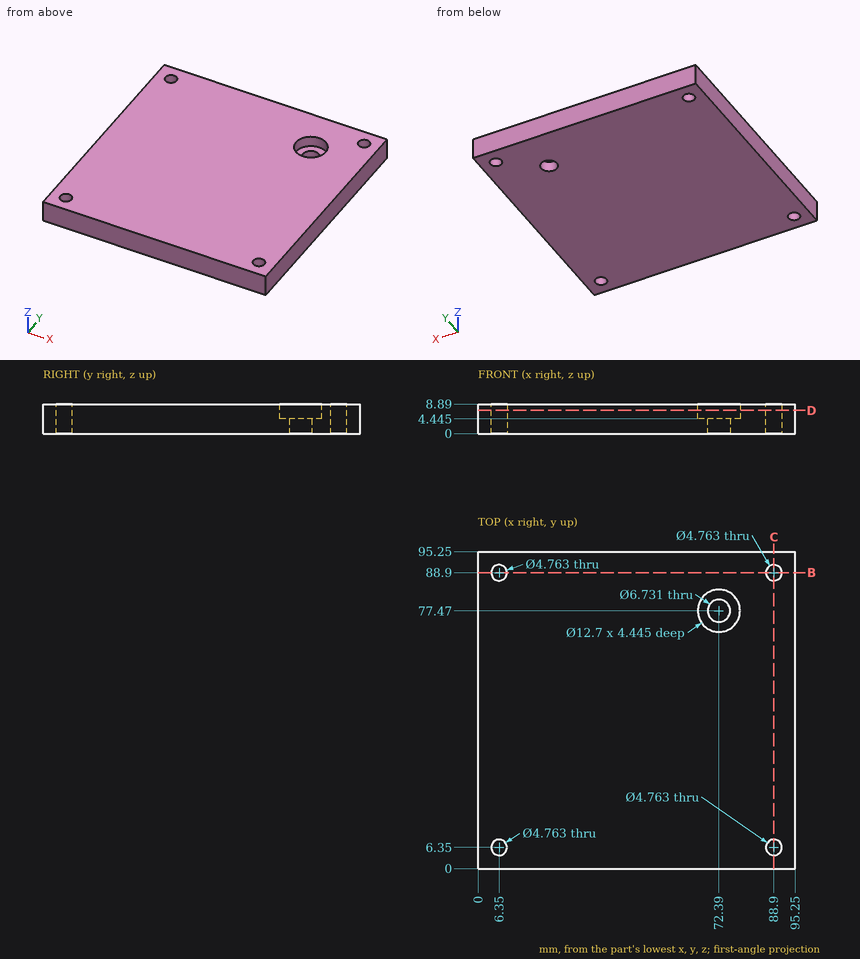
Source: three-view drawing plus pictorial views. Frame: mm from the lowest corner of the part. Coordinates: 2 decimals unless noted, no trailing zeros. Loops run counter-clockwise (first coordinate to the right, second up) from the corner with the lowest first, then second, coordinate; pieces in that order, holes last. Notation, with made-up numbers: (-13.5, 71) - (7.5, 71) arc R23 cw to (7.5, 96) - close; hole circle Ø6 at (-22.75, 4.25). An arc over 180 degrees is marked (long way). One line per item, written item: value. Start each with the question number.
1. Section B-B (y = 88.9). Return the cut outline in (x, z).
2. Ray query, L1, parallel to Y at x = 88.9, z = 7; L2, parallel to X at y = 7, z = 8; L3, parallel to Y at x = 88.5, z = 8. Return the intervals inside material, ascending.
3. Section D-D (z = 7). Return the cut outline in (x, y).
4. Contact query for flat-ended pins moving along their axis: P1, Ø4, axis at x = 72.39, y = 77.47, coming from the +Z side; P2, Ø4, axis at x = 75, y = 75.5, coming from the +Z side (1 decimal). Output: stop coordinate, or through.
Verdict:
1. outline: (0, 0) - (3.97, 0) - (3.97, 8.89) - (0, 8.89) - close; (8.73, 0) - (86.52, 0) - (86.52, 8.89) - (8.73, 8.89) - close; (91.28, 0) - (95.25, 0) - (95.25, 8.89) - (91.28, 8.89) - close
2. L1: y = 0 to 3.97, 8.73 to 86.52, 91.28 to 95.25
2. L2: x = 0 to 4.06, 8.64 to 86.61, 91.19 to 95.25
2. L3: y = 0 to 4, 8.7 to 86.55, 91.25 to 95.25
3. outline: (0, 0) - (95.25, 0) - (95.25, 95.25) - (0, 95.25) - close; hole circle Ø4.76 at (6.35, 6.35); hole circle Ø4.76 at (6.35, 88.9); hole circle Ø12.7 at (72.39, 77.47); hole circle Ø4.76 at (88.9, 6.35); hole circle Ø4.76 at (88.9, 88.9)
4. P1: passes through
4. P2: stops at z = 4.4
